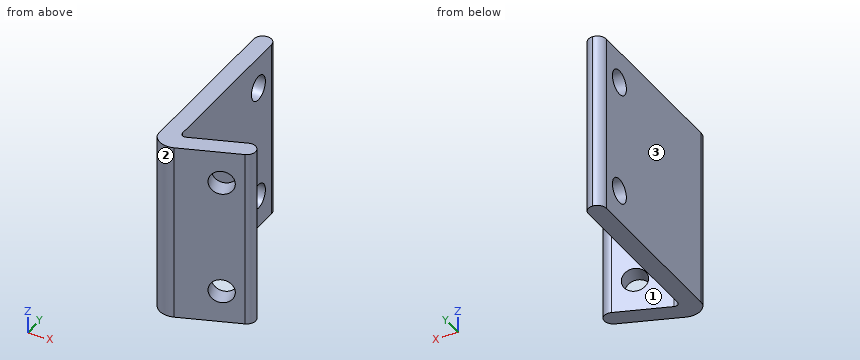
from build123d import *

# Parameters (mm, degrees)
SKETCH3_W           = 20
SKETCH3_H           = 10
SKETCH3_R           = 1.35
BOSS_EXTRUDE1_DEPTH = 2
SKETCH2_W           = 20
SKETCH2_H           = 20
SKETCH2_R           = 1.375
BOSS_EXTRUDE2_DEPTH = 2
FILLET1_R           = 2
FILLET2_R           = 0.5
FILLET3_R           = 1
FILLET4_R           = 1


# Some blends are built 0.0001 mm under size
with BuildPart() as part:
    # Sketch3 → Boss-Extrude1 (new body)
    with BuildSketch(Plane(origin=(0, 0, 0), x_dir=(0, 0, -1), z_dir=(0.34202014332566616, -0.9396926207859094, 0))):
        with Locations((10, 5)):
            Rectangle(SKETCH3_W, SKETCH3_H)
        with Locations(Location((3.6, 6.69633816, 0), (0, 0, 90))):
            Circle(SKETCH3_R, mode=Mode.SUBTRACT)
        with Locations(Location((16.4, 6.69633816, 0), (0, 0, 90))):
            Circle(SKETCH3_R, mode=Mode.SUBTRACT)
    extrude(amount=BOSS_EXTRUDE1_DEPTH)

    # Sketch2 → Boss-Extrude2 (add)
    with BuildSketch(Plane(origin=(0, 0, 0), x_dir=(0, 0, -1), z_dir=(1, 0, 0))):
        with Locations((10, 10)):
            Rectangle(SKETCH2_W, SKETCH2_H)
        with Locations((3.597100601, 16.415608196)):
            Circle(SKETCH2_R, mode=Mode.SUBTRACT)
        with Locations((16.397100601, 16.415608196)):
            Circle(SKETCH2_R, mode=Mode.SUBTRACT)
    extrude(amount=BOSS_EXTRUDE2_DEPTH)

    # Fillet1
    # the kernel refuses this fillet: 2 mm, written as the material it takes off along each edge
    with BuildSketch(Plane(origin=(0.684040287, -1.879385242, -25), x_dir=(0.9396926207859093, 0.34202014332566616, 0), z_dir=(0, 0, 1))) as fillet1_piece_1:
        with BuildLine():
            CenterArc((FILLET1_R, FILLET1_R), FILLET1_R, 180, 90)
            Line((0, FILLET1_R), (0, 0))
            Line((0, 0), (FILLET1_R, 0))
        make_face()
    extrude(amount=30, mode=Mode.SUBTRACT)
    with BuildSketch(Plane(origin=(0, 0, -20.881634904), x_dir=(0.34202014332566616, -0.9396926207859093, 0), z_dir=(0, 0, 1))) as fillet1_piece_2:
        with BuildLine():
            CenterArc((FILLET1_R * 0.176326980708, FILLET1_R), FILLET1_R, 250, 20)
            Line((-FILLET1_R * 0.165693162617, FILLET1_R * 0.0603073792141), (0, 0))
            Line((0, 0), (FILLET1_R * 0.176326980708, 0))
        make_face()
    extrude(amount=21.763269807, mode=Mode.SUBTRACT)

    # Fillet2
    fillet2_edges = [part.edges().sort_by_distance(p)[0] for p in [
        (2, 0.727940469, -10),
    ]]
    fillet(fillet2_edges, radius=FILLET2_R)

    # Fillet3
    fillet3_edges = [part.edges().sort_by_distance(p)[0] for p in [
        (2, 20, -10),
        (0, 20, -10),
    ]]
    fillet(fillet3_edges, radius=FILLET3_R - 0.0001)  # a hair under: the kernel refuses the full size

    # Fillet4
    fillet4_edges = [part.edges().sort_by_distance(p)[0] for p in [
        (10.080966495, 1.540816192, -10),
        (9.396926208, 3.420201433, -10),
    ]]
    fillet(fillet4_edges, radius=FILLET4_R - 0.0001)  # a hair under: the kernel refuses the full size


solid = part.part
Source: CAD feature listing. Evaluate the final solid. Frame: model axes, mm. Face numbers are marked on the shaded views. Give positions to 0.01 mm unless a question says otherwise; leave off trailing zeros. Write each loop counter-clockwise with the first axis right and the second up, starting at its lowest first coordinate (ties: lowest second). Pieces come first, ordered by that corner, then holes. Notation, with made-up numbers: (-5, 3.25) -> (19, 3.25) arc R17 ccw to (19, 9.25) -> close; hole circle Ø4 at (69.5, -17). An arc over 180 degrees is marked (long way). Write item = value, one per line.
Q1. First-contact query: pin 1 (2.5 mm diameter, centred on y = 16.42, z = -16.4, fed in from +X); pin 2 (3.5 mm diameter, centred on y = 16.42, z = -3.6, fed in from +X); pin 3 (1 mm diameter, centred on x = 5.5, z = -16.5, fed in from -Y); pin 4 (3 mm diameter, centred on x = 6, z = -15, fed in from +Y). Flat tips, straight axial feed; report the tip coordinate or a pass-through.
Here are the results:
pin_1 = through
pin_2 = 2
pin_3 = -0.31
pin_4 = 2.73
Q2. Cut plane A-A on z = -16.75. State how many separate pieces and enclosed holes the cut face has, then the cut area to 3 significant figures.
Here are the results:
separate_pieces = 3
enclosed_holes = 0
area = 47.1 mm²
Q3. Cut plane B-B on y = 17.25. Return loops of the section in (x, z), then the cut area to 3 significant figures.
Here are the results:
outline = (0, -20) -> (2, -20) -> (2, -17.49) -> (0, -17.49) -> close; (0, -15.3) -> (2, -15.3) -> (2, -4.69) -> (0, -4.69) -> close; (0, -2.5) -> (2, -2.5) -> (2, 0) -> (0, 0) -> close
area = 31.3 mm²
Q4. Line query: line 1 (X direction, y = 14.25, z = -18.5); line 2 (Y direction, x = 2.75, z = -12.5); line 3 (Y direction, x = 4.25, z = -19). Output: solid intervals per line, ascending. Write a range as from..to.
Here are the results:
line_1 = 0..2
line_2 = -1.13..1
line_3 = -0.58..1.55
Q5. Mould query, pull axis X, two halves, no side actions, for the marked faces 1, 2 and 3. Classes: +X half, -X half, draft (parallel to the pull), parting line (faces both ways), or undercut.
Here are the results:
face_1 = undercut
face_2 = parting line
face_3 = -X half
